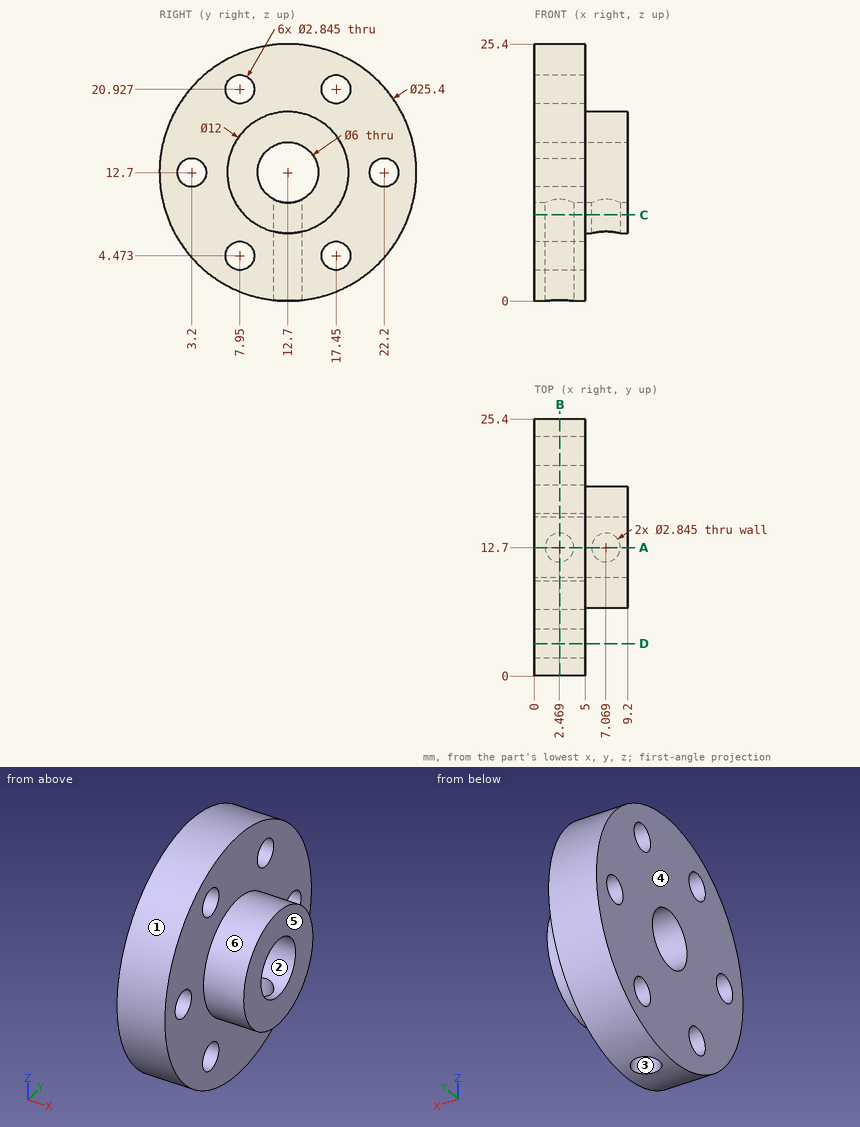
Can you work these out from the drawing? Everything is in mm from the part's minimum corner. A direction names the side the tool comes from. Coordinates: 2 decimals unless noted, no trailing zeros. Loops run counter-clockwise (first coordinate to the right, second up) from the corner with the lowest first, then second, coordinate; pieces in that order, holes last.
1. For P1, Ø1.7, axis at y = 17.45, z = 4.47, coming from the +X side; P2, Ø1.5, axis at x = 2, y = 15, coming from the +Z side (3 decimals); P3, Ø3.5, axis at y = 17.45, z = 20.93, coming from the +X side; P4, Ø5, axis at x = 4.5, z = 6, coming from the -Y side (1 decimal), each with a flat end and sliding along its axis, tell me the tip position at first contact or that it passes through.
2. I need wall thicknesses on L1, parallel to Y at x = 1.85, z = 12.7; L2, parallel to X at y = 2.75, z = 10.75; L3, parallel to Y at x = 5.75, z = 12.7. Which ranges of each line are inside material? Lowest first, please.
3. Imagine slicing it at A-A, the plane y = 12.7. Please give me the cut outline in (x, z).
4. Imagine slicing it at D-D, the plane y = 3.2. Please give me the cut outline in (x, z).
5. Imagine slicing it at C-C, the plane z = 8.5. Please give me the cut outline in (x, y) (1 decimal).
6. If we mould it in two halves opening along Y, with no side actions, what happens to the marked faces 1, 2, 3 and 4? For each: pulls with the +Y half, pulls with the -Y half, needs draft (parallel to the pull), parting line crosses it, or undercut.
7. Imagine slicing it at B-B, the plane x = 2.5. Count the separate pieces of the cut face and the enclosed holes in it.
8. For the marked faces 5 and 6, which set-ups out of +Z, -Z, +X, -X, +Y, -Y let a thin tool reach every point of the face, with its end or its side?
Taken from the geometry:
1. P1: passes through
1. P2: stops at z = 25.305
1. P3: stops at x = 5
1. P4: stops at y = 0.7
2. L1: y = 0 to 1.78, 4.62 to 9.7, 15.7 to 20.78, 23.62 to 25.4
2. L2: x = 0 to 5
2. L3: y = 6.7 to 9.7, 15.7 to 18.7
3. outline: (0, 0) - (1.05, 0) - (1.05, 9.7) - (0, 9.7) - close; (0, 15.7) - (9.2, 15.7) - (9.2, 18.7) - (5, 18.7) - (5, 25.4) - (0, 25.4) - close; (3.89, 0) - (5, 0) - (5, 6.7) - (5.65, 6.7) - (5.65, 9.7) - (3.89, 9.7) - close; (8.49, 6.7) - (9.2, 6.7) - (9.2, 9.7) - (8.49, 9.7) - close
4. outline: (0, 4.27) - (5, 4.27) - (5, 11.28) - (0, 11.28) - close; (0, 14.12) - (5, 14.12) - (5, 21.13) - (0, 21.13) - close
5. outline: (0, 0.7) - (5, 0.7) - (5, 8.4) - (9.2, 8.4) - (9.2, 17) - (5, 17) - (5, 24.7) - (0, 24.7) - close; hole circle Ø2.8 at (2.5, 12.7); hole circle Ø2.8 at (7.1, 12.7)
6. face 1: parting line crosses it
6. face 2: undercut
6. face 3: undercut
6. face 4: needs draft
7. separate pieces: 1
7. enclosed holes: 6
8. face 5: +Z, -Z, +X, +Y, -Y
8. face 6: +X
